Verification items for the finished model (mm, model axes). Round coordinates to 2 decimals unless told otherwise and drop trailing zeros. Write each loop counter-clockwise with the first axis right and the second up, starting at its lowest first coordinate (ties: lowest second). Pieces come first, ordered by that corner, then holes. Notation, with made-up numbers: M -30,-10.75 L -21,-10.75 A37 cw -21,28.25 Z; hole C 73.5,-20 d9. An arc over 180 degrees is marked long. Answer in a Markdown table with one row per item. Add a question column.
1. Sectioned sample at D-D on x = 6. Record the cut outline in (y, z), plus the area to 3 significant figures.
2. Sectioned sample at C-C on y = 2.05. Record the cut outline in (x, z), plus the area to 3 significant figures.
3. Sectioned sample at A-A on x = 19.5. Record the cut outline in (y, z), plus the area to 3 significant figures.
4. Material ranges on probe 1 along Z at (x, y) = (16, 0.8); probe 2 along Z at (x, y) = (6, 3.15); probe 3 along X at (y, z) = (0.4, 50), recorded low to high.
5. Draft check along X on faces 1 (the flat face through (30, 2, 50)), 2 (the flat face through (16, 2, 26)), 3 (the cylindrical face through (5.675, 2.028, 37.536)). Enter one of: pulls with the +X half, pulls with the -X half, needs draft (parallel to the pull), parting line crosses it, or undercut.
6. Sectioned sample at B-B on z = 50.5. Record the cut outline in (x, y).
```python
from build123d import *

# Parameters (mm, degrees)
CYLINDER879_R     = 12.5
CYLINDER879_DEPTH = 10
CYLINDER877_R     = 1.5
CYLINDER877_DEPTH = 10
CYLINDER878_R     = 1.5
CYLINDER878_DEPTH = 10
BOX424_W          = 28
BOX424_H          = 4
BOX424_DEPTH      = 48


with BuildPart() as obj1:
    # Cylinder879 → Cylinder879 (new body)
    with BuildSketch(Plane(origin=(16, 7, 50.5), x_dir=(1, 0, 0), z_dir=(0, -1, 0))):
        Circle(CYLINDER879_R)
    extrude(amount=CYLINDER879_DEPTH)


with BuildPart() as obj2:
    # Cylinder877 → Cylinder877 (new body)
    with BuildSketch(Plane(origin=(29, 6, 63), x_dir=(1, 0, 0), z_dir=(0, -1, 0))):
        Circle(CYLINDER877_R)
    extrude(amount=CYLINDER877_DEPTH)


with BuildPart() as compound504:
    # Cylinder878 → Cylinder878 (new body)
    with BuildSketch(Plane(origin=(10, 6, 39), x_dir=(1, 0, 0), z_dir=(0, -1, 0))):
        Circle(CYLINDER878_R)
    extrude(amount=CYLINDER878_DEPTH)

    # Compound504: union obj2
    add(obj2.part)


with BuildPart() as compound504_1:
    # Compound504 placement: moved
    add(compound504.part.moved(Location((-4, 0, 0))))


with BuildPart() as cut022:
    # Box424 → Box424 (new body)
    with BuildSketch(Plane(origin=(2, 0, 26), x_dir=(1, 0, 0), z_dir=(0, 0, 1))):
        with Locations((14, 2)):
            Rectangle(BOX424_W, BOX424_H)
    extrude(amount=BOX424_DEPTH)

    # Cut021: cut Compound504
    add(compound504_1.part, mode=Mode.SUBTRACT)

    # Cut022: cut obj1
    add(obj1.part, mode=Mode.SUBTRACT)


solid = cut022.part
```
Geometry check:
| question | item | result |
|---|---|---|
| 1 | outline | M 0,26 L 4,26 L 4,37.5 L 0,37.5 Z; M 0,40.5 L 4,40.5 L 4,43 L 0,43 Z; M 0,58 L 4,58 L 4,74 L 0,74 Z |
| 1 | area | 120 mm2 |
| 2 | outline | M 2,26 L 30,26 L 30,74 L 2,74 Z; hole C 16,50.5 d25; hole C 6,39 d3; hole C 25,63 d3 |
| 2 | area | 839 mm2 |
| 3 | outline | M 0,26 L 4,26 L 4,38.5 L 0,38.5 Z; M 0,62.5 L 4,62.5 L 4,74 L 0,74 Z |
| 3 | area | 96.0 mm2 |
| 4 | probe 1 | z = 26 to 38, 63 to 74 |
| 4 | probe 2 | z = 26 to 37.5, 40.5 to 43, 58 to 74 |
| 4 | probe 3 | x = 2 to 3.51, 28.49 to 30 |
| 5 | face 1 | pulls with the +X half |
| 5 | face 2 | needs draft |
| 5 | face 3 | undercut |
| 6 | outline | M 2,0 L 3.5,0 L 3.5,4 L 2,4 Z; M 28.5,0 L 30,0 L 30,4 L 28.5,4 Z |
